Geometry check sheet. Reference: the model listing, model coordinates, mm. A direction names the side the tool comes from. Round coordinates to 2 decimals unless told otherwise and drop trailing zeros. Write each loop counter-clockwise with the first axis right and the second up, starting at its lowest first coordinate (ties: lowest second). Pieces come first, ordered by that corner, then holes. Notation, with made-up numbers: (26.25, -6) -> (40.25, -6) arc R16 cw to (40.25, 8) -> close; hole circle Ø10 at (18.5, 75). An arc over 180 degrees is marked (long way). Return JSON: item names as keys, results as strings. Group by question number.
from build123d import *

# Parameters (mm, degrees)
F0_R     = 75
F1_DEPTH = 5
F2_R     = 75
F2_R_2   = 70
F3_DEPTH = 300
F5_DEPTH = 250
F6_R     = 1.5
F7_DEPTH = 25
F9_DEPTH = 10


with BuildPart() as f1:
    # F0 (on Top) → F1 (new body)
    with BuildSketch(Plane.XY):
        Circle(F0_R)
    extrude(amount=F1_DEPTH)

    # F2 (on face) → F3 (join)
    with BuildSketch(Plane.XY.offset(5)):
        Circle(F2_R)
        Circle(F2_R_2, mode=Mode.SUBTRACT)
    extrude(amount=F3_DEPTH)

    # F4 (on face) → F5 (cut)
    with BuildSketch(Plane.XY.offset(305)):
        with BuildLine():
            Line((25, -70.7106781187), (25, -65.3834841531))
            ThreePointArc((25, -65.3834841531), (0, -70), (-25, -65.3834841531))
            Line((-25, -65.3834841531), (-25, -70.7106781187))
            ThreePointArc((-25, -70.7106781187), (0, -75), (25, -70.7106781187))
        make_face()
    extrude(amount=-F5_DEPTH, mode=Mode.SUBTRACT)

    # F6 (on face) → F7 (cut)
    with BuildSketch(Plane.XY.offset(5)):
        with Locations((-15.5, 60.5)):
            Circle(F6_R)
        with BuildLine():
            ThreePointArc((17, 60.5), (15.5, 62), (14, 60.5))
            ThreePointArc((14, 60.5), (15.5, 59), (17, 60.5))
        make_face()
        with BuildLine():
            ThreePointArc((17, 29.5), (15.5, 31), (14, 29.5))
            ThreePointArc((14, 29.5), (15.5, 28), (17, 29.5))
        make_face()
        with Locations((-15.5, 29.5)):
            Circle(F6_R)
    extrude(amount=-F7_DEPTH, mode=Mode.SUBTRACT)

    # F8 (on face) → F9 (join)
    with BuildSketch(Plane.XY.offset(5)):
        with BuildLine():
            ThreePointArc((-40.1313972081, -27.5), (-40.386953511, -25.5588571617), (-41.1362066798, -23.75))
            ThreePointArc((-41.1362066798, -23.75), (-54.8758409053, -29.4411428383), (-40.1313972081, -27.5))
        make_face()
        with BuildLine():
            ThreePointArc((-42.6313972081, -27.5), (-52.4610263396, -28.7940952255), (-43.3012701892, -25))
            ThreePointArc((-43.3012701892, -25), (-42.8017680767, -26.2059047745), (-42.6313972081, -27.5))
        make_face(mode=Mode.SUBTRACT)
        with BuildLine():
            ThreePointArc((55.1313972081, -27.5), (49.5725400464, -20.2555563028), (41.1362066798, -23.75))
            ThreePointArc((41.1362066798, -23.75), (45.6902543699, -34.7444436972), (55.1313972081, -27.5))
        make_face()
        with BuildLine():
            ThreePointArc((52.6313972081, -27.5), (46.3373019826, -32.3296291314), (43.3012701892, -25))
            ThreePointArc((43.3012701892, -25), (48.9254924337, -22.6703708686), (52.6313972081, -27.5))
        make_face(mode=Mode.SUBTRACT)
    extrude(amount=F9_DEPTH)


solid = f1.part
1) Mould release check, pull along X, two halves, no side actions. Record for faces 4 (the face through (-9.764, 74.362, 150.365)), 5 (the face through (-1, 1, 0)), 6 (the face through (37.632, 59.024, 152.9)), 7 (the face through (53, -29, 15)): +X half, -X half, draft (parallel to the pull), parting line (faces both ways), or undercut.
2) Sectioned sample at C-C on z = 21. Enter the section's corners in (x, y).
3) Sectioned sample at A-A on x = 0. Enter the section's corners in (y, z).
4) Sectioned sample at B-B on y = 19. Enter the section's corners in (x, z), and give its area (3 significant figures).
5) Material ranges on probe 1 along Z at (x, y) = (-25, 11.5); probe 2 along X at (y, z) = (-16.5, 123); probe 3 along X at (y, z) = (-36.5, 40), recorded low to high. Write a range as [from, to].
6) Tool access check on faces 1 (the face through (48, -27, 5)), 2 (the face through (0, -71, 55)), 3 (the face through (33, 62, 305)). Record the directions out of +Z, -Z, +X, -X, +Y, -Y that give a thin tool (end or side, any length) a straight path to the whole face; none if there is none.
7) Go/stop test with flat-tipped pins: P1, Ø3, axis at x = -7.5, y = -72, coming from the +Z side; P2, Ø3, axis at x = -46.5, y = -29, coming from the +Z side; P3, Ø8, axis at y = 48, z = 265, coming from the -X side. Record where each tip stops, or that it passes through.
8) Sectioned sample at D-D on z = 220. Enter the section's corners in (x, y).
Evaluation:
{
 "1": {"face 4": "parting line", "face 5": "draft", "face 6": "undercut", "face 7": "undercut"},
 "2": {"outline": "circle Ø150 at (0, 0); hole circle Ø140 at (0, 0)"},
 "3": {"outline": "(-75, 0) -> (75, 0) -> (75, 305) -> (70, 305) -> (70, 5) -> (-70, 5) -> (-70, 55) -> (-75, 55) -> close"},
 "4": {"outline": "(-72.55, 0) -> (72.55, 0) -> (72.55, 305) -> (67.37, 305) -> (67.37, 5) -> (-67.37, 5) -> (-67.37, 305) -> (-72.55, 305) -> close", "area": "3,830 mm2"},
 "5": {"probe 1": "z = [0, 5]", "probe 2": "x = [-73.16, -68.03], [68.03, 73.16]", "probe 3": "x = [-65.52, -59.73], [59.73, 65.52]"},
 "6": {"face 1": "+Z", "face 2": "+Z, -Y", "face 3": "+Z, +X, -X, +Y, -Y"},
 "7": {"P1": "stops at z = 55", "P2": "stops at z = 5", "P3": "stops at x = -60.74"},
 "8": {"outline": "(-25, -70.71) -> (-25, -65.38) arc R70 cw (long way) to (25, -65.38) -> (25, -70.71) arc R75 ccw (long way) to start"}
}
